Geometry check sheet. Reference: the model listing, model coordinates, mm. A direction names the side the tool comes from. Round coordinates to 2 decimals unless told otherwise and drop trailing zeros. Order: outer loops, then holes, each group sorted by start corner. A loop starts at its lowest first (then second) coordinate and runs counter-clockwise, first axis right, second up. Notation, with made-up numbers: (5, 89.5) - (17, 89.5) arc R12 cw to (17, 93.5) - close; hole circle Ø3 at (67.5, 76.5). An arc over 180 degrees is marked (long way). Use a Markdown table: item, result. Add a question column.
(1) Mould release check, pull along Y, two halves, no side actions. Record for faces 4 (the face through (-0.05, -70.46, 4.44)), 5 (the face through (14.52, -23.81, 4.44)), 6 (the face through (-8, -12, 0)): released by +Y, released by -Y, zero draft, split by the parting line, or undercut.
(2) Section check A-A on z = 3. Record the boundary of the cut face in (x, y).
(3) Section check C-C on y = -14. Record the boundary of the cut face in (x, z).
(4) Thickness scan on line 1 along Y through (x, z) = (0, 2.25); line 2 along Y through (x, z) = (-1, 5.5); line 3 along X through (y, z) = (-26.5, 0.5). Record the ranges inside material, lowest first. Write a range as [from, to].
(5) Section check B-B on x = 0. Record the boundary of the cut face in (y, z), then the cut area to 3 significant figures.
(6) Gauge pin test, flat ends, axial feed: P1, Ø1.5, axis at y = -1, z = 3.5, coming from the +X side; P2, Ø4, axis at x = 5.5, z = 6, coming from the +Y side; P3, Ø2, axis at y = 2, z = 6.5, coming from the -X side. Record the tip position at first contact, or that the pin passes through.
(7) Section check D-D on x = -10.5. Record the boundary of the cut face in (y, z).
(8) Access from +Z, -Z, +X, -X, +Y, -Y to the whole of each face (thin tool, end or side, straight path). Record for faces 1 (the face through (-14.49, -27.22, 4.44)), 2 (the face through (10.195, 10.14, 4.437)), 3 (the face through (13.187, 9.678, 4.437)).
```python
from build123d import *

# Parameters (mm, degrees)
EXTRUDE_1_DEPTH = 9


with BuildPart() as part:
    # 草图1 → 凸台-拉伸1 (new body)
    with BuildSketch(Plane.XY):
        with BuildLine():
            Line((9, -4.461217091), (20.194287223, -43.700074535))
            ThreePointArc((20.194287223, -43.700074535), (-0.601689007, -70.452595567), (-19.831131739, -42.552800924))
            Line((-19.831131739, -42.552800924), (-9, -11.461217091))
            Line((-9, -11.461217091), (-17.512781831, 24.379158821))
            ThreePointArc((-17.512781831, 24.379158821), (0.492386715, 46.532047075), (17.259086335, 23.427624637))
            Line((17.259086335, 23.427624637), (9, -4.461217091))
        make_face()
        with BuildLine():
            Line((-14.593984859, 25.072429503), (-6.081203028, -10.767946409))
            ThreePointArc((-6.081203028, -10.767946409), (-6.003901946, -11.614176084), (-6.16698118, -12.448133686))
            Line((-6.16698118, -12.448133686), (-16.998112919, -43.539717519))
            ThreePointArc((-16.998112919, -43.539717519), (-0.515733435, -67.453827213), (17.309389049, -44.5230949))
            Line((17.309389049, -44.5230949), (6.115101825, -5.284237456))
            ThreePointArc((6.115101825, -5.284237456), (6.000037583, -4.446200468), (6.123485611, -3.609357379))
            Line((6.123485611, -3.609357379), (14.382571946, 24.279484349))
            ThreePointArc((14.382571946, 24.279484349), (0.410322262, 43.533169714), (-14.593984859, 25.072429503))
        make_face(mode=Mode.SUBTRACT)
    extrude(amount=EXTRUDE_1_DEPTH)


solid = part.part
```
Check sheet entries:
| question | item | result |
|---|---|---|
| 1 | face 4 | split by the parting line |
| 1 | face 5 | undercut |
| 1 | face 6 | zero draft |
| 2 | outline | (-19.83, -42.55) arc R21 ccw (long way) to (20.19, -43.7) - (9, -4.46) - (17.26, 23.43) arc R18 ccw (long way) to (-17.51, 24.38) - (-9, -11.46) - close; hole (-17, -43.54) arc R18 ccw (long way) to (17.31, -44.52) - (6.12, -5.28) arc R3 cw to (6.12, -3.61) - (14.38, 24.28) arc R15 ccw (long way) to (-14.59, 25.07) - (-6.08, -10.77) arc R3 cw to (-6.17, -12.45) - close |
| 3 | outline | (-9.88, 0) - (-6.71, 0) - (-6.71, 9) - (-9.88, 9) - close; (8.6, 0) - (11.72, 0) - (11.72, 9) - (8.6, 9) - close |
| 4 | line 1 | y = [-70.46, -67.46], [43.54, 46.54] |
| 4 | line 2 | y = [-70.44, -67.43], [43.51, 46.51] |
| 4 | line 3 | x = [-14.24, -11.06], [12.17, 15.29] |
| 5 | outline | (-70.46, 0) - (-67.46, 0) - (-67.46, 9) - (-70.46, 9) - close; (43.54, 0) - (46.54, 0) - (46.54, 9) - (43.54, 9) - close |
| 5 | area | 54.0 mm2 |
| 6 | P1 | stops at x = 10.25 |
| 6 | P2 | stops at y = 46.2 |
| 6 | P3 | stops at x = -12.43 |
| 7 | outline | (-67.65, 0) - (-64.08, 0) - (-64.08, 9) - (-67.65, 9) - close; (-24.89, 0) - (-15.77, 0) - (-15.77, 9) - (-24.89, 9) - close; (-5.15, 0) - (7.84, 0) - (7.84, 9) - (-5.15, 9) - close; (39.25, 0) - (43.16, 0) - (43.16, 9) - (39.25, 9) - close |
| 8 | face 1 | +Z, -Z, -X |
| 8 | face 2 | +Z, -Z |
| 8 | face 3 | +Z, -Z, +X |
